CAD build for the part. Positions are in the model's coordinates, mm. Round coordinates to 2 decimals unless told otherwise and drop trailing zeros. Loops run counter-clockwise (first coordinate to the right, second up) from the corner with the lowest first, then second, coordinate; pieces in that order, holes last. Notation, with made-up numbers: (-11.75, -25.75) -> (1.25, -25.75) arc R10 ccw to (1.25, -21.75) -> close; hole circle Ø10 at (88.5, 20.5). An arc over 180 degrees is marked (long way). Answer as CSV lines item,"result".
```python
from build123d import *

# Parameters (mm, degrees)
F1_DEPTH = 6


with BuildPart() as f1:
    # F0 (on Top) → F1 (new body)
    with BuildSketch(Plane.XY):
        Polygon((-33.457938, -5.590482), (-40.954886, 1.906467), (-40.954886, -48.093533), (9.045114, -48.093533), align=None)
        Polygon((-25.954887, 1.911273), (-40.954886, 1.906467), (-33.457938, -5.590482), align=None)
        Polygon((-25.954887, 1.911273), (-33.457938, -5.590482), (9.045114, -48.093533), (9.043877, -33.093533), align=None)
    extrude(amount=F1_DEPTH)


solid = f1.part
```
Q1. Slice it at B-B, the plane x = -8. Give the cut face in (y, z), and give its area (3 significant figures).
Results:
outline,"(-48.09, 0) -> (-16.05, 0) -> (-16.05, 6) -> (-48.09, 6) -> close"
area,"192 mm2"
Q2. Drop flat-ended pins along their axis: pin 1 Ø3 at (x, z) = (-37, 3) entering from +Y; pin 2 Ø10 at (x, y) = (-12.5, -3.5) entering from +Z. Give the stop position or say it passes through.
Results:
pin 1,"y = 1.91"
pin 2,"through"
Q3. Slice it at C-C, the plane y = -26. Give the cut face in (x, z).
Results:
outline,"(-40.95, 0) -> (1.95, 0) -> (1.95, 6) -> (-40.95, 6) -> close"
Q4. Probe L1, parallel to Y at x = -35, z = 5.75; L2, parallel to Y at x = -25.5, z = 4.55; L3, parallel to X at y = -20, z = 3.8. List the from-to ranges inside material, lowest first. Write a range as [from, to].
Results:
L1,"[-48.09, 1.91]"
L2,"[-48.09, 1.46]"
L3,"[-40.95, -4.05]"
Q5. Slice it at A-A, the plane z = 2. Give the cut face in (x, y), and give its area (3 significant figures).
Results:
outline,"(-40.95, -48.09) -> (9.05, -48.09) -> (9.04, -33.09) -> (-25.95, 1.91) -> (-40.95, 1.91) -> close"
area,"1,890 mm2"
